Work out the finished part from the listing and answer in its coordinate system (mm). A direction names the side the tool comes from. Coordinates: 2 decimals unless noted, no trailing zeros. Loops run counter-clockwise (first coordinate to the right, second up) from the corner with the lowest first, then second, coordinate; pieces in that order, holes last. Notation, with made-up numbers: (58.5, 9) -> (69.5, 9) arc R12 ccw to (69.5, 25) -> close; hole circle Ø6 at (24, -22.75). An arc over 180 degrees is marked (long way). Use a Markdown table: item, result.
from build123d import *

# Parameters (mm, degrees)
F1_DEPTH = 8
F2_R     = 7.8
F2_R_2   = 6.8
F3_DEPTH = 7
F4_R     = 1.65
F5_DEPTH = 8.2775166443
F6_R     = 1.65
F7_DEPTH = 9.3042205827


with BuildPart() as f1:
    # F0 (on Front) → F1 (new body)
    with BuildSketch(Plane.XZ):
        with BuildLine():
            Line((20.9, 0), (4, 0))
            ThreePointArc((4, 0), (1.1715728753, -1.1715728753), (0, -4))
            Line((0, -4), (0, -45.9))
            ThreePointArc((0, -45.9), (1.1715728753, -48.7284271247), (4, -49.9))
            Line((4, -49.9), (20.9, -49.9))
            ThreePointArc((20.9, -49.9), (23.7284271247, -48.7284271247), (24.9, -45.9))
            Line((24.9, -45.9), (24.9, -4))
            ThreePointArc((24.9, -4), (23.7284271247, -1.1715728753), (20.9, 0))
        make_face()
    extrude(amount=F1_DEPTH)

    # F2 (on face) → F3 (cut)
    with BuildSketch(Plane.XZ.offset(8)):
        with Locations((9, -9)):
            Circle(F2_R)
        with Locations((15.9, -24)):
            Circle(F2_R_2)
        with Locations((9, -39)):
            Circle(F2_R)
    extrude(amount=-F3_DEPTH, mode=Mode.SUBTRACT)

    # F4 (on face) → F5 (cut, through all)
    with BuildSketch(Plane.YZ.offset(24.9)):
        with Locations((-4, -39)):
            Circle(F4_R)
        with Locations((-4, -9)):
            Circle(F4_R)
    extrude(amount=-F5_DEPTH, mode=Mode.SUBTRACT)

    # F6 (on face) → F7 (cut, through all)
    with BuildSketch(Plane(origin=(0, 0, 0), x_dir=(0, -1, 0), z_dir=(-1, 0, 0))):
        with Locations((4, -24)):
            Circle(F6_R)
    extrude(amount=-F7_DEPTH, mode=Mode.SUBTRACT)


solid = f1.part
Q1. For faces 1 (the flat face through (12, 0, -25)), 2 (the cylindrical face through (20.82, -5.65, -8.93)), 3 (the flat face through (9, -1, -9)), 4 (the cylindrical face through (4.586, -3.785, -22.364)), determine the directions among +Z, -Z, +X, -X, +Y, -Y from which every point of the face is accessible in a straight line to the end or side of a thin tool.
Solved:
| item | result |
|---|---|
| face 1 | +Z, -Z, +X, -X, +Y |
| face 2 | +X |
| face 3 | -Y |
| face 4 | -X |
Q2. Section A-A on z = -39 is taken. Determine the outline of the cut face in (x, y).
Solved:
| item | result |
|---|---|
| outline | (0, -8) -> (1.2, -8) -> (1.2, -1) -> (16.8, -1) -> (16.8, -2.35) -> (24.9, -2.35) -> (24.9, 0) -> (0, 0) -> close; (16.8, -8) -> (24.9, -8) -> (24.9, -5.65) -> (16.8, -5.65) -> close |
Q3. Section B-B on y = -1.75 is taken. Determine the outline of the cut face in (x, z).
Solved:
| item | result |
|---|---|
| outline | (0, -45.9) arc R4 ccw to (4, -49.9) -> (20.9, -49.9) arc R4 ccw to (24.9, -45.9) -> (24.9, -4) arc R4 ccw to (20.9, 0) -> (4, 0) arc R4 ccw to (0, -4) -> close; hole circle Ø15.6 at (9, -39); hole circle Ø15.6 at (9, -9); hole circle Ø13.6 at (15.9, -24) |
Q4. Consider line 1 (Y direction, x = 18.5, z = -9); line 2 (Z direction, x = 8.25, y = -7); line 3 (Z direction, x = 8, y = -5.25). Determine where each line is inside the solid, lowest interval first. Write a range as [from, to].
Solved:
| item | result |
|---|---|
| line 1 | [-8, -5.65], [-2.35, 0] |
| line 2 | [-49.9, -46.76], [-31.24, -16.76], [-1.24, 0] |
| line 3 | [-49.9, -46.74], [-31.26, -25.08], [-22.92, -16.74], [-1.26, 0] |
Q5. Determine the mould class of faces 5 (the flat face through (16, -1, -24)), 6 (the cylindrical face through (23.759, -3.944, -1.203)), 7 (the flat face through (13, -4, 0)), 8 (the flat face through (9, -1, -39)) for opening direction X: pulls with the +X half, pulls with the -X half, needs draft (parallel to the pull), parting line crosses it, or undercut.
Solved:
| item | result |
|---|---|
| face 5 | undercut |
| face 6 | pulls with the +X half |
| face 7 | needs draft |
| face 8 | undercut |
Q6. Section D-D on z = -18 is taken. Determine the outline of the cut face in (x, y).
Solved:
| item | result |
|---|---|
| outline | (0, -8) -> (12.7, -8) -> (12.7, -1) -> (19.1, -1) -> (19.1, -8) -> (24.9, -8) -> (24.9, 0) -> (0, 0) -> close |
Q7. Given pin 1 Ø8 at (x, z) = (8.5, -37.5) entering from -Y, flat-ended and moving along its own axis, determine where the tip first touches the part or whether it passes through.
Solved:
| item | result |
|---|---|
| pin 1 | y = -1 |
Q8. Section C-C on x = 3.25 is taken. Determine the outline of the cut face in (y, z).
Solved:
| item | result |
|---|---|
| outline | (-8, -49.83) -> (0, -49.83) -> (0, -0.07) -> (-8, -0.07) -> (-8, -3.73) -> (-1, -3.73) -> (-1, -14.27) -> (-8, -14.27) -> (-8, -33.73) -> (-1, -33.73) -> (-1, -44.27) -> (-8, -44.27) -> close; hole circle Ø3.3 at (-4, -24) |
